Here's how the part is built. I have some questions about the finished solid (model axes, mm). Give positions to 0.01 mm unless a question says otherwise; leave off trailing zeros. Loops run counter-clockwise (first coordinate to the right, second up) from the corner with the lowest first, then second, coordinate; pieces in that order, holes last. Notation, with made-up numbers: (-9, 87) - (-5, 87) arc R26 cw to (-5, 115) - close; hole circle Ø5 at (67.5, 17.5). An arc over 180 degrees is marked (long way). Use a Markdown table: item, result.
from build123d import *

# Parameters (mm, degrees)
SKETCH_1_R      = 2.2
EXTRUDE_1_DEPTH = 5


with BuildPart() as part:
    # 草图1 → 凸台-拉伸1 (new body)
    with BuildSketch(Plane.XY):
        Polygon((-200, 150), (200, 150), (200, 110), (205, 110), (205, 70), (200, 70), (200, 30), (205, 30), (205, -30), (200, -30), (200, -70), (205, -70), (205, -110), (200, -110), (200, -150), (160, -150), (160, -155), (120, -155), (120, -150), (80, -150), (80, -155), (40, -155), (40, -150), (-40, -150), (-40, -155), (-80, -155), (-80, -150), (-120, -150), (-120, -155), (-160, -155), (-160, -150), (-200, -150), (-200, -110), (-205, -110), (-205, -70), (-200, -70), (-200, -30), (-205, -30), (-205, 30), (-200, 30), (-200, 70), (-205, 70), (-205, 110), (-200, 110), align=None)
        with Locations((-140, -140)):
            Circle(SKETCH_1_R, mode=Mode.SUBTRACT)
        with Locations((-100, -140)):
            Circle(SKETCH_1_R, mode=Mode.SUBTRACT)
        with Locations((-60, -140)):
            Circle(SKETCH_1_R, mode=Mode.SUBTRACT)
        with Locations((-20, -140)):
            Circle(SKETCH_1_R, mode=Mode.SUBTRACT)
        with Locations((20, -140)):
            Circle(SKETCH_1_R, mode=Mode.SUBTRACT)
        with Locations((60, -140)):
            Circle(SKETCH_1_R, mode=Mode.SUBTRACT)
        with Locations((100, -140)):
            Circle(SKETCH_1_R, mode=Mode.SUBTRACT)
        with Locations((140, -140)):
            Circle(SKETCH_1_R, mode=Mode.SUBTRACT)
        with Locations((-190, 110)):
            Circle(SKETCH_1_R, mode=Mode.SUBTRACT)
        with Locations((-190, 70)):
            Circle(SKETCH_1_R, mode=Mode.SUBTRACT)
        with Locations((-190, 30)):
            Circle(SKETCH_1_R, mode=Mode.SUBTRACT)
        with Locations((-190, -30)):
            Circle(SKETCH_1_R, mode=Mode.SUBTRACT)
        with Locations((-190, -70)):
            Circle(SKETCH_1_R, mode=Mode.SUBTRACT)
        with Locations((-190, -110)):
            Circle(SKETCH_1_R, mode=Mode.SUBTRACT)
        with Locations((190, -110)):
            Circle(SKETCH_1_R, mode=Mode.SUBTRACT)
        with Locations((190, -70)):
            Circle(SKETCH_1_R, mode=Mode.SUBTRACT)
        with Locations((190, -30)):
            Circle(SKETCH_1_R, mode=Mode.SUBTRACT)
        with Locations((190, 30)):
            Circle(SKETCH_1_R, mode=Mode.SUBTRACT)
        with Locations((190, 70)):
            Circle(SKETCH_1_R, mode=Mode.SUBTRACT)
        with Locations((190, 110)):
            Circle(SKETCH_1_R, mode=Mode.SUBTRACT)
    extrude(amount=EXTRUDE_1_DEPTH)


solid = part.part
(1) Will these pins go through, and if not, where does the flat tip stop? pin 1 (2.5 mm diameter, centred on y = 52.5, z = 3, fed in from +X); pin 2 (2.5 mm diameter, centred on y = 129.5, z = 2, fed in from -X); pin 3 (1.5 mm diameter, centred on x = -179.5, z = 3, fed in from -Y); pin 4 (5 mm diameter, centred on x = -190, y = 70, fed in from -Z).
A:
| item | result |
|---|---|
| pin 1 | x = 200 |
| pin 2 | x = -200 |
| pin 3 | y = -150 |
| pin 4 | z = 0 |
(2) If I drill on line 1 (Y direction, x = 140, z = 1.15); line 2 (X direction, y = -115, z = 2.55), over which ranges is the centre line in solid material (lowest first)?
A:
| item | result |
|---|---|
| line 1 | -155 to -142.2, -137.8 to 150 |
| line 2 | -200 to 200 |
(3) Suppose I cut it at A-A on y = -117.5. Write out the boundary of the cut face in (x, z).
A:
| item | result |
|---|---|
| outline | (-200, 0) - (200, 0) - (200, 5) - (-200, 5) - close |
